Read the model definition and answer for the solid it produces. Units are mm, in the model's axes. Face numbers are marked on the shaded views. Round coordinates to 2 decimals unless told otherwise and drop trailing zeros. Write each loop counter-clockwise with the first axis right and the second up, starting at its lowest first coordinate (ties: lowest second). Pieces come first, ordered by that corner, then holes. Notation, with made-up numbers: (71.5, 14.5) -> (130.5, 14.5) arc R9 ccw to (130.5, 24.5) -> close; hole circle Ø11 at (-5, 11.25). An arc over 180 degrees is marked (long way). Return JSON: item names as keys, results as strings. Group by question number.
(1) A cutting plane is placed at A-A on y = 0. Give the vertices of the cut face in (x, z).
(2) A cutting plane is placed at B-B on x = 0. Give the vertices of the cut face in (y, z).
(3) The mould has two halves that part along Y. Classify the marked faces 1, 2 and 3: released by +Y, released by -Y, zero draft, split by the parting line, or undercut.
(4) A cutting plane is placed at C-C on z = 13.75. Give the vertices of the cut face in (x, y).
(5) Given pin 1 (2 mm diameter, centred on x = 7, y = -10.5, fed in from -Z); pin 2 (12 mm diameter, centred on x = 11, z = 4, fed in from +Y); pin 3 (1 mm diameter, centred on y = -8, z = 17, fed in from +X); pin 4 (3 mm diameter, centred on y = -3, z = 12.5, fed in from +X), each flat-ended and moving along its own axis, determine where each tip first touches the part or whether it passes through.
(6) Straight lines are drawn through the part: line 1 (Y direction, x = 0, z = 12.5); line 2 (X direction, y = -5.5, z = 9); line 3 (Y direction, x = -11.75, z = 2.75). For each, find the intervals that lie inside material, in ascending order.
(7) A cutting plane is placed at D-D on y = -12. Give the vertices of the cut face in (x, z), then the cut area to 3 significant figures.
```python
from build123d import *

# Parameters (mm, degrees)
SKETCH1_R           = 15
BOSS_EXTRUDE1_DEPTH = 20
SKETCH2_R           = 5
SKETCH2_R_2         = 2
CUT_EXTRUDE1_DEPTH  = 30.154759474


with BuildPart() as part:
    # Sketch1 → Boss-Extrude1 (new body)
    with BuildSketch(Plane.XY):
        Circle(SKETCH1_R)
    extrude(amount=BOSS_EXTRUDE1_DEPTH)

    # Sketch2 → Cut-Extrude1 (cut, through all)
    with BuildSketch(Plane.XY.offset(20)):
        Circle(SKETCH2_R)
        with Locations((0, 12)):
            Circle(SKETCH2_R_2)
        with Locations((10.392304845, 6)):
            Circle(SKETCH2_R_2)
        with Locations((10.392304845, -6)):
            Circle(SKETCH2_R_2)
        with Locations((0, -12)):
            Circle(SKETCH2_R_2)
        with Locations((-10.392304845, -6)):
            Circle(SKETCH2_R_2)
        with Locations((-10.392304845, 6)):
            Circle(SKETCH2_R_2)
    extrude(amount=-CUT_EXTRUDE1_DEPTH, mode=Mode.SUBTRACT)


solid = part.part
```
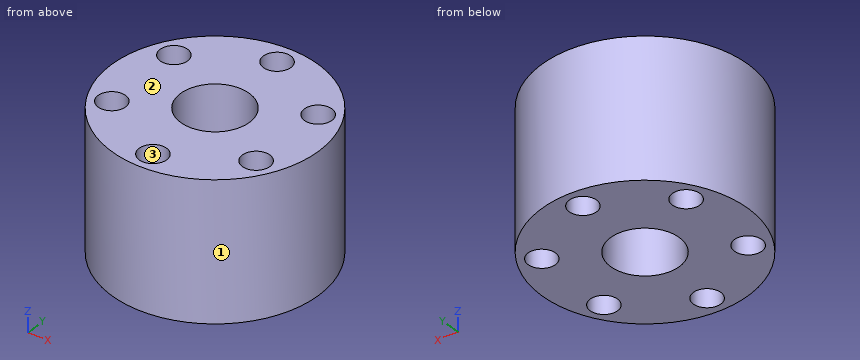
Checks:
{
 "1": {"outline": "(-15, 0) -> (-5, 0) -> (-5, 20) -> (-15, 20) -> close; (5, 0) -> (15, 0) -> (15, 20) -> (5, 20) -> close"},
 "2": {"outline": "(-15, 0) -> (-14, 0) -> (-14, 20) -> (-15, 20) -> close; (-10, 0) -> (-5, 0) -> (-5, 20) -> (-10, 20) -> close; (5, 0) -> (10, 0) -> (10, 20) -> (5, 20) -> close; (14, 0) -> (15, 0) -> (15, 20) -> (14, 20) -> close"},
 "3": {"face 1": "split by the parting line", "face 2": "zero draft", "face 3": "undercut"},
 "4": {"outline": "circle Ø30 at (0, 0); hole circle Ø4 at (-10.39, -6); hole circle Ø4 at (-10.39, 6); hole circle Ø10 at (0, 0); hole circle Ø4 at (0, -12); hole circle Ø4 at (0, 12); hole circle Ø4 at (10.39, -6); hole circle Ø4 at (10.39, 6)"},
 "5": {"pin 1": "stops at z = 0", "pin 2": "stops at y = 14.14", "pin 3": "stops at x = 12.99", "pin 4": "stops at x = 14.92"},
 "6": {"line 1": "y = -15 to -14, -10 to -5, 5 to 10, 14 to 15", "line 2": "x = -13.96 to -12.33, -8.46 to 8.46, 12.33 to 13.96", "line 3": "y = -9.32 to -7.47, -4.53 to 4.53, 7.47 to 9.32"},
 "7": {"outline": "(-9, 0) -> (-2, 0) -> (-2, 20) -> (-9, 20) -> close; (2, 0) -> (9, 0) -> (9, 20) -> (2, 20) -> close", "area": "280 mm^2"}
}
